Can you work these out from the model? Positions are in its coordinate system, mm. Coordinates: 2 decimals unless noted, no trailing zeros. Order: outer loops, then holes, each group sorted by start corner. A loop starts at its lowest first (then second) coordinate and runs counter-clockwise, first axis right, second up. Notation, with made-up numbers: (-32, 71) -> (19, 71) arc R34 ccw to (19, 109) -> close; hole circle Ø8 at (-4.75, 88). An arc over 180 degrees is marked (long way). Return JSON: item names as keys, results as strings. Group by question number.
1) For pin 1 (8 mm diameter, centred on x = 9.5, z = 215.5, fed in from -Y); pin 2 (5.5 mm diameter, centred on x = 12.7, z = 584.2, fed in from +Y), each with a flat end and sliding along its axis, tell me the tip position at first contact or that it passes through.
2) If I drill on probe 1 along X at (y, z) = (0.55, 584.2) (3 decimals); probe 2 along Y at (x, z) = (9, 126), over which ranges is the centre line in solid material (lowest first)? Write a range as from..to.
3) If we section it at C-C, the plane z = 417.5: Please give me the cut outline in (x, y), then the cut area to 3 significant figures.
4) If we section it at A-A, the plane z = 341: Please give me the cut outline in (x, y).
5) If we section it at B-B, the plane x = 19.75: Please give me the cut outline in (y, z).
Autodesk Inventor part; units mm, degrees
ref_plane "YZ Plane" through (0, 0, 0) normal (1, 0, 0) x (0, 1, 0)
ref_plane "XZ Plane" through (0, 0, 0) normal (0, 1, 0) x (-1, 0, 0)
ref_plane "XY Plane" through (0, 0, 0) normal (0, 0, 1) x (1, 0, 0)
sketch "Sketch1" plane through (0, 0, 0) normal (0, 0, 1) x (1, 0, 0)
  line L0 (0, 0) -> (25.4, 0)
  line L1 (25.4, 0) -> (25.4, 25.4)
  line L2 (25.4, 25.4) -> (0, 25.4)
  line L3 (0, 25.4) -> (0, 0)
  line L4 (1.5875, 23.8125) -> (23.8125, 23.8125)
  line L5 (23.8125, 23.8125) -> (23.8125, 1.5875)
  line L6 (23.8125, 1.5875) -> (1.5875, 1.5875)
  line L7 (1.5875, 1.5875) -> (1.5875, 23.8125)
  dimension "d0" = 25.4
  dimension "d1" = 25.4
  dimension "d2" = 1.5875
extrude "Extrusion1" add sketch "Sketch1" along normal blind 596.9
sketch "Sketch2" plane through (0, 0, 0) normal (-1, 0, 0) x (0, 0, 1)
  line L0 (0, 25.4) -> (0, 0)
  line L1 (0, 0) -> (596.9, 0)
  line L2 (596.9, 25.4) -> (596.9, 0)
  line L3 (0, 25.4) -> (596.9, 25.4)
  line L4 (25.4, 16.8275) -> (381, 16.8275)
  arc A0 (381, 13.6525) -> (381, 16.8275) centre (381, 15.24) ccw
  line L5 (381, 13.6525) -> (25.4, 13.6525)
  arc A1 (25.4, 16.8275) -> (25.4, 13.6525) centre (25.4, 15.24) ccw
  dimension "d5" = 3.175
  dimension "d6" = 355.6
  dimension "d9" = 10.16
  dimension "d24" = 25.4
extrude "Extrusion2" cut sketch "Sketch2" against normal through all contours L4 A0 L5 A1
sketch "Sketch3" plane through (0, 25.4, 0) normal (0, 1, 0) x (1, 0, 0)
  line L0 (25.4, 0) -> (0, 0)
  line L1 (0, 0) -> (0, -596.9)
  line L2 (25.4, -596.9) -> (0, -596.9)
  line L3 (25.4, 0) -> (25.4, -596.9)
  point P0 (0, 0)
  point P1 (12.7, -584.2)
  dimension "d13" = 12.7
  dimension "d14" = 12.7
  dimension "d23" = 12.7
hole "Hole1" at (12.7, 25.4, 584.2) direction (0, -1, 0) diameter 6.35 end through all
properties part number "ScissorLiftBase"
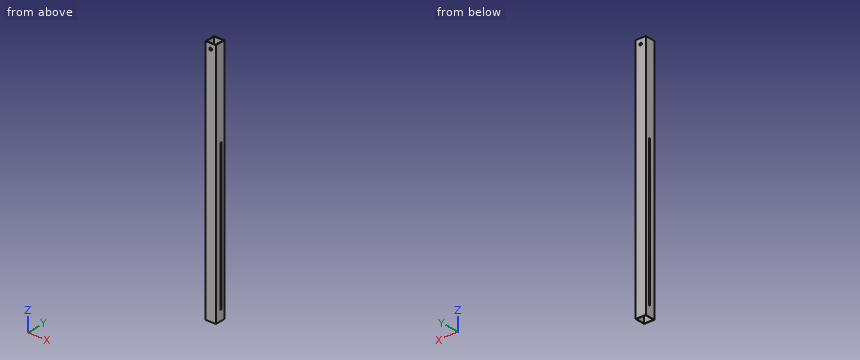
Result sheet:
{
 "1": {"pin 1": "stops at y = 0", "pin 2": "passes through"},
 "2": {"probe 1": "x = 0..9.525, 15.875..25.4", "probe 2": "y = 0..1.59, 23.81..25.4"},
 "3": {"outline": "(0, 0) -> (25.4, 0) -> (25.4, 25.4) -> (0, 25.4) -> close; hole (1.59, 1.59) -> (23.81, 1.59) -> (23.81, 23.81) -> (1.59, 23.81) -> close", "area": "151 mm2"},
 "4": {"outline": "(0, 0) -> (25.4, 0) -> (25.4, 13.65) -> (23.81, 13.65) -> (23.81, 1.59) -> (1.59, 1.59) -> (1.59, 13.65) -> (0, 13.65) -> close; (0, 16.83) -> (1.59, 16.83) -> (1.59, 23.81) -> (23.81, 23.81) -> (23.81, 16.83) -> (25.4, 16.83) -> (25.4, 25.4) -> (0, 25.4) -> close"},
 "5": {"outline": "(0, 0) -> (1.59, 0) -> (1.59, 596.9) -> (0, 596.9) -> close; (23.81, 0) -> (25.4, 0) -> (25.4, 596.9) -> (23.81, 596.9) -> close"}
}
